```python
from build123d import *

# Parameters (mm, degrees)
SKETCH2_W           = 55
SKETCH2_H           = 12
BOSS_EXTRUDE1_DEPTH = 6
SKETCH3_W           = 25
SKETCH3_H           = 12
BOSS_EXTRUDE2_DEPTH = 13
SKETCH4_R           = 4
CUT_EXTRUDE2_DEPTH  = 30
SKETCH5_W           = 20.513890507
SKETCH5_H           = 7
CUT_EXTRUDE3_DEPTH  = 5
SKETCH6_R           = 1.6
CUT_EXTRUDE4_DEPTH  = 11
CUT_EXTRUDE5_DEPTH  = 3
SKETCH8_R           = 0.75
CUT_EXTRUDE6_DEPTH  = 3


with BuildPart() as part:
    # Sketch2 → Boss-Extrude1 (new body)
    with BuildSketch(Plane.XY):
        with Locations((27.5, 6)):
            Rectangle(SKETCH2_W, SKETCH2_H)
        with BuildLine():
            Line((6.5, 8.5), (9.5, 8.5))
            ThreePointArc((9.5, 8.5), (12, 6), (9.5, 3.5))
            Line((9.5, 3.5), (6.5, 3.5))
            ThreePointArc((6.5, 3.5), (4, 6), (6.5, 8.5))
        make_face(mode=Mode.SUBTRACT)
        with BuildLine():
            Line((48.5, 8.5), (45.5, 8.5))
            ThreePointArc((45.5, 8.5), (43, 6), (45.5, 3.5))
            Line((45.5, 3.5), (48.5, 3.5))
            ThreePointArc((48.5, 3.5), (51, 6), (48.5, 8.5))
        make_face(mode=Mode.SUBTRACT)
    extrude(amount=BOSS_EXTRUDE1_DEPTH)

    # Sketch3 → Boss-Extrude2 (add)
    with BuildSketch(Plane.XY.offset(6)):
        with Locations((27.5, 6)):
            Rectangle(SKETCH3_W, SKETCH3_H)
    extrude(amount=BOSS_EXTRUDE2_DEPTH)

    # Sketch4 → Cut-Extrude2 (cut)
    with BuildSketch(Plane.XZ):
        with BuildLine():
            ThreePointArc((28.127016654, 10), (28, 11), (28.127016654, 12))
            Line((28.127016654, 12), (15, 12))
            Line((15, 12), (15, 10))
            Line((15, 10), (28.127016654, 10))
        make_face()
        with Locations((32, 11)):
            Circle(SKETCH4_R)
    extrude(amount=-CUT_EXTRUDE2_DEPTH, mode=Mode.SUBTRACT)

    # Sketch5 → Cut-Extrude3 (cut)
    with BuildSketch(Plane(origin=(0, 0, 0), x_dir=(-1, 0, 0), z_dir=(0, 0, -1))):
        with Locations((-27.415473723, 6)):
            Rectangle(SKETCH5_W, SKETCH5_H)
    extrude(amount=-CUT_EXTRUDE3_DEPTH, mode=Mode.SUBTRACT)

    # Sketch6 → Cut-Extrude4 (cut)
    with BuildSketch(Plane.XY.offset(19)):
        with Locations((21, 6)):
            Circle(SKETCH6_R)
    extrude(amount=-CUT_EXTRUDE4_DEPTH, mode=Mode.SUBTRACT)

    # Sketch7 → Cut-Extrude5 (cut)
    with BuildSketch(Plane(origin=(0, 0, 5), x_dir=(-1, 0, 0), z_dir=(0, 0, -1))):
        Polygon((-17.535898385, 6), (-19.267949192, 9), (-22.732050808, 9), (-24.464101615, 6), (-22.732050808, 3), (-19.267949192, 3), align=None)
    extrude(amount=-CUT_EXTRUDE5_DEPTH, mode=Mode.SUBTRACT)

    # Sketch8 → Cut-Extrude6 (cut)
    with BuildSketch(Plane.XY.offset(19)):
        with Locations((36.85, 8)):
            Circle(SKETCH8_R)
        with Locations((30.35, 8)):
            Circle(SKETCH8_R)
    extrude(amount=-CUT_EXTRUDE6_DEPTH, mode=Mode.SUBTRACT)


solid = part.part
```
Could you check a few things on this model? Use its own coordinates, in mm. A direction names the side the tool comes from. Give positions to 0.01 mm unless a question says otherwise; leave off trailing zeros. Order: outer loops, then holes, each group sorted by start corner. A loop starts at its lowest first (then second) coordinate and runs counter-clockwise, first axis right, second up.
Q1. For faces 1 (the cylindrical face through (12, 6, 3)), 2 (the flat face through (40, 6, 12)), 3 (the flat face through (15, 6, 15)), 4 (the flat face through (21, 9, 6)), which set-ups out of +Z, -Z, +X, -X, +Y, -Y let a thin tool reach every point of the face, with its end or its side?
Q2. Suppose I cut it at A-A, the plane x = 21. Write out the boundary of the cut face in (y, z), and give its area (3 significant figures).
Q3. If I drill on line 1 along Y through (x, z) = (31, 2.75); line 2 along Y through (x, z) = (5, 3.25); line 3 along Z through (x, y) = (20, 4.5), over which ranges is the centre line in solid material (lowest first)?
Q4. We'd pull the mould along Y, two halves only. Please class faces 5 (the cylindrical face through (37.196, 7.335, 17.521)), 6 (the flat face through (47, 8.5, 3)), 7 (the flat face through (47, 9, 6)): +Y half, -Y half, draft (parallel to the pull), parting line (faces both ways), or undercut.
Q5. Suppose I cut it at D-D, the plane x = 32. Write out the boundary of the cut face in (y, z).
Q6. Suppose I cut it at C-C, the plane y = 11.25. Write out the boundary of the cut face in (x, z).
Q7. I'm going to push flat-ended pins straight in: P1, Ø2.5, axis at x = 21, y = 6, coming from the -Z side; P2, Ø5.5, axis at x = 32, y = 7.5, coming from the -Z side; P3, Ø4, axis at y = 3.5, z = 13.5, coming from the -X side; P4, Ø2, axis at x = 11, y = 7, coming from the +Z side. Where does each tip first touch, or does it pass through?
Q8. Suppose I cut it at B-B, the plane z = 13.5. Write out the boundary of the cut face in (x, y), and give its area (3 significant figures).
Solution:
1. face 1: +Z, -Z
1. face 2: +Z, +X, +Y, -Y
1. face 3: +Z, -X, +Y, -Y
1. face 4: -Z
2. outline: (0, 0) - (2.5, 0) - (2.5, 5) - (3, 5) - (3, 8) - (4.4, 8) - (4.4, 10) - (0, 10) - close; (0, 12) - (4.4, 12) - (4.4, 19) - (0, 19) - close; (7.6, 8) - (9, 8) - (9, 5) - (9.5, 5) - (9.5, 0) - (12, 0) - (12, 10) - (7.6, 10) - close; (7.6, 12) - (12, 12) - (12, 19) - (7.6, 19) - close
2. area: 122 mm2
3. line 1: y = 0 to 2.5, 9.5 to 12
3. line 2: y = 0 to 4, 8 to 12
3. line 3: z = 8 to 10, 12 to 19
4. face 5: undercut
4. face 6: undercut
4. face 7: draft
5. outline: (0, 0) - (2.5, 0) - (2.5, 5) - (9.5, 5) - (9.5, 0) - (12, 0) - (12, 7) - (0, 7) - close; (0, 15) - (12, 15) - (12, 19) - (0, 19) - close
6. outline: (0, 0) - (55, 0) - (55, 6) - (40, 6) - (40, 19) - (15, 19) - (15, 12) - (28.13, 12) arc R4 cw (long way) to (28.13, 10) - (15, 10) - (15, 6) - (0, 6) - close
7. P1: passes through
7. P2: stops at z = 0
7. P3: stops at x = 15
7. P4: stops at z = 6
8. outline: (15, 0) - (28.88, 0) - (28.88, 12) - (15, 12) - close; (35.12, 0) - (40, 0) - (40, 12) - (35.12, 12) - close; hole circle Ø3.2 at (21, 6)
8. area: 217 mm2
